Autodesk Inventor part; units mm, degrees
ref_plane "YZ Plane" through (0, 0, 0) normal (1, 0, 0) x (0, 1, 0)
ref_plane "XZ Plane" through (0, 0, 0) normal (0, 1, 0) x (-1, 0, 0)
ref_plane "XY Plane" through (0, 0, 0) normal (0, 0, 1) x (1, 0, 0)
sketch "Sketch1" plane through (0, 0, 0) normal (0, 0, 1) x (1, 0, 0)
  line L0 (0, 0) -> (380, 0)
  line L1 (380, 0) -> (380, 124)
  line L2 (380, 124) -> (179, 124)
  line L3 (179, 124) -> (179, 184)
  line L4 (179, 184) -> (0, 184)
  line L5 (0, 184) -> (0, 0)
  dimension "d0" = 380
  dimension "d1" = 124
  dimension "d2" = 201
  dimension "d3" = 60
extrude "Extrusion1" add sketch "Sketch1" along normal blind 3
sketch "Sketch2" plane through (0, 0, 3) normal (0, 0, 1) x (1, 0, 0)
  line L0 (0, 184) -> (0, 0)
  line L1 (179, 184) -> (0, 184)
  line L2 (0, 0) -> (380, 0)
  line L3 (380, 0) -> (380, 124)
  line L4 (380, 124) -> (179, 124)
  point P0 (20, 20)
  point P1 (20, 164)
  point P2 (360, 104)
  point P3 (360, 20)
  dimension "d6" = 20
  dimension "d7" = 20
  dimension "d8" = 20
  dimension "d9" = 20
  dimension "d10" = 20
  dimension "d11" = 20
  dimension "d12" = 20
  dimension "d13" = 20
hole "Hole1" at (20, 20, 3) at (20, 164, 3) at (360, 104, 3) at (360, 20, 3) direction (0, 0, -1) diameter 7 end through all
sketch "Sketch3" plane through (0, 0, 3) normal (0, 0, 1) x (1, 0, 0)
  line L0 (0, 0) -> (380, 0)
  line L1 (0, 184) -> (0, 0)
  point P0 (153.17, 121.31)
  point P1 (226.83, 121.31)
  dimension "d21" = 73.66
  dimension "d22" = 121.31
  dimension "d23" = 121.31
  dimension "d24" = 153.17
hole "Hole2" at (153.17, 121.31, 3) at (226.83, 121.31, 3) direction (0, 0, -1) diameter 3.5 end through all
sketch "Sketch4" plane through (380, 0, 0) normal (1, 0, 0) x (0, 0, -1)
  line L0 (0, 124) -> (-3, 124)
  line L1 (0, 0) -> (-3, 0)
  line L2 (-3, 0) -> (-3, 124)
  line L3 (-3, 124) -> (0, 124)
  line L4 (0, 124) -> (0, 0)
extrude "Extrusion2" add sketch "Sketch4" along normal blind 26
sketch "Sketch5" plane through (0, 0, 3) normal (0, 0, 1) x (1, 0, 0)
  circle A0 centre (241.7805, 9.3195) radius 2.5
  circle A1 centre (175.7805, 60.3195) radius 2.5
  circle A2 centre (254.2805, 116.8195) radius 2.5
  circle A3 centre (79.2805, 116.8195) radius 2.5
  circle A4 centre (89.2805, 6.8195) radius 2.5
  line L0 (179, 124) -> (406, 124)
  line L1 (179, 184) -> (0, 184)
  line L2 (0, 184) -> (0, 0)
  dimension "d65" = 7.1805
  dimension "d66" = 7.1805
  dimension "d67" = 67.1805
  dimension "d68" = 114.6805
  dimension "d69" = 63.6805
  dimension "d70" = 117.1805
  dimension "d71" = 177.1805
  dimension "d72" = 79.2805
  dimension "d73" = 89.2805
  dimension "d74" = 175.7805
  dimension "d75" = 241.7805
  dimension "d76" = 254.2805
hole "Hole3" at (241.7805, 9.3195, 3) at (254.2805, 116.8195, 3) at (175.7805, 60.3195, 3) at (89.2805, 6.8195, 3) at (79.2805, 116.8195, 3) direction (0, 0, -1) diameter 3.242 depth 5 tip angle 118
sketch "Sketch6" plane through (0, 0, 3) normal (0, 0, 1) x (1, 0, 0)
  circle A0 centre (225.65, 120.31) radius 1.75
  circle A1 centre (151.99, 120.31) radius 1.75
  point P0 (0, 0)
hole "Hole4" at (225.65, 120.31, 3) at (151.99, 120.31, 3) direction (0, 0, -1) diameter 3 depth 5 tip angle 118
sketch "Sketch7" plane through (0, 0, 3) normal (0, 0, 1) x (1, 0, 0)
  circle A0 centre (151.99, 120.31) radius 1.75
  circle A1 centre (225.65, 120.31) radius 1.75
  line L0 (179, 124) -> (406, 124)
  line L1 (0, 184) -> (0, 0)
  point P0 (228.19, 34.585)
  point P1 (148.18, 34.585)
  dimension "d48" = 85.725
  dimension "d49" = 85.725
  dimension "d50" = 80.01
  dimension "d51" = 2.54
  dimension "d52" = 3.69
  dimension "d53" = 89.415
  dimension "d54" = 151.99
  dimension "d55" = 148.18
  dimension "d56" = 73.66
  dimension "d57" = 228.19
hole "Hole5" at (228.19, 34.585, 3) at (148.18, 34.585, 3) direction (0, 0, -1) diameter 2.5 depth 5 tip angle 118
properties part number "SupportsheetEPS" material "Aluminum 6061"
Design review of the part built by this model. Coordinates are the model's own, in mm. Coordinates: 2 decimals unless noted, no trailing zeros. Order: outer loops, then holes, each group sorted by start corner. A loop starts at its lowest first (then second) coordinate and runs counter-clockwise, first axis right, second up. Notation, with made-up numbers: (4.25, -34.5) -> (15.25, -34.5) arc R10 ccw to (15.25, -22.5) -> close; hole circle Ø9 at (-22.75, 82.25). An arc over 180 degrees is marked (long way). Use one line per item in the form item = value. Start each with the question number.
(1) Add section C-C on y = 141.5. State the section outline as (x, z) points.
(2) Add section B-B on x = 247. State the section outline as (y, z) points, plus the area to 3 significant figures.
(3) For probe 1 along X at (y, z) = (164, 1.5); probe 2 along X at (y, z) = (133.5, 1.95); probe 3 along Y at (x, z) = (79, 0.65), list the stretches that pass through material, from the lowest coordinate up.
(4) Add section A-A on z = 1.65. Give the number of separate pieces and of enclosed holes in the cut face, plus the area to 3 significant figures.
(5) Insertion check: pin 1 (0.9 mm diameter, centred on x = 239.5, z = 2, fed in from +Y); pin 2 (1.9 mm diameter, centred on x = 89.28, y = 6.82, fed in from +Z); pin 3 (4 mm diameter, centred on x = 228.19, y = 34.585, fed in from +Z). Each pin has a flat end and moves straight along its axis. Give the tip position at first contact, or say it passes through.
(6) The part is to be moulded in two halves that separate along Y. For faces 1 (the flat face through (200, 70, 3)), 2 (the cylindrical face through (363.105, 18.385, 1.479)), say which applies: +Y half, -Y half, draft (parallel to the pull), parting line (faces both ways), or undercut.
Answer block:
q1.outline = (0, 0) -> (179, 0) -> (179, 3) -> (0, 3) -> close
q2.outline = (0, 0) -> (124, 0) -> (124, 3) -> (0, 3) -> close
q2.area = 372 mm²
q3.probe_1 = 0 to 16.5, 23.5 to 179
q3.probe_2 = 0 to 179
q3.probe_3 = 0 to 115.22, 118.42 to 184
q4.separate_pieces = 1
q4.enclosed_holes = 13
q4.area = 60,900 mm²
q5.pin_1 = 124
q5.pin_2 = through
q5.pin_3 = 3
q6.face_1 = draft
q6.face_2 = undercut
